Model file for the job. Use its own axes, mm. Face numbers are marked on the shaded views. A direction names the side the tool comes from. Round coordinates to 2 decimals unless told otherwise and drop trailing zeros. Loops run counter-clockwise (first coordinate to the right, second up) from the corner with the lowest first, then second, coordinate; pieces in that order, holes last. Notation, with made-up numbers: M -13.5,15.25 L 27.5,15.25 A24 cw 27.5,44.25 Z; hole C 4,50.25 d2. An arc over 180 degrees is marked long. Use a Markdown table: item, result. Add a question column.
Item 1: Saw through at D-D on z = 3.25. Write the cut outline in (x, y).
Item 2: Tool access for the marked faces 1, 2, 3, 4 and 5: list every direction of +Z, -Z, +X, -X, +Y, -Y with a clear straight run to the whole face (end or side of a thin tool).
Item 3: Wall check: L1, parallel to Y at x = -1.25, z = 0; L2, parallel to Y at x = 3, z = 0; L3, parallel to Z at x = 5, y = -4.25. Give the ranges that are in metal, low to high. Write a range as from..to.
Item 4: Saw through at A-A on z = 0. Write the cut outline in (x, y).
Item 5: Two-plate mould, pull along Y, no slides. Class the marked faces 6, 7 and 8: +Y half, -Y half, draft (parallel to the pull), parting line (faces both ways), or undercut.
Item 6: Saw through at B-B on y = 0. Write the cut outline in (x, z).
Item 7: Pin check, flat tips, straight feed: P1, Ø3, axis at y = -2, z = 7, coming from the -X side; P2, Ø6, axis at x = -1.5, z = 4, coming from the -Y side; P3, Ø6, axis at x = -4.5, y = -0.5, coming from the -Z side. Stop position of each tip, or through.
Item 8: Saw through at C-C on x = 9.25. Write the cut outline in (y, z).
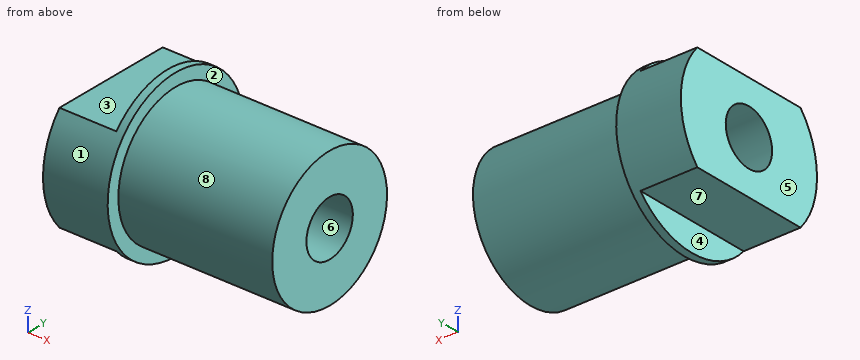
```python
from build123d import *

# Parameters (mm, degrees)
SKETCH2_R               = 7.9375
BOSS_EXTRUDE1_DEPTH     = 6.35
SKETCH3_R               = 6.6929
BOSS_EXTRUDE2_DEPTH     = 15.113
SKETCH4_W               = 5.588
SKETCH4_H               = 2.76225
CUT_EXTRUDE1_DEPTH      = 6.35
F_1_4_28_TAPPED_HOLE1_D = 5.4102


with BuildPart() as part:
    # Sketch2 → Boss-Extrude1 (new body)
    with BuildSketch(Plane(origin=(0, 0, 0), x_dir=(0, 0, -1), z_dir=(1, 0, 0))):
        Circle(SKETCH2_R)
    extrude(amount=-BOSS_EXTRUDE1_DEPTH)

    # Sketch3 → Boss-Extrude2 (add)
    with BuildSketch(Plane(origin=(0, 0, 0), x_dir=(0, 0, -1), z_dir=(1, 0, 0))):
        Circle(SKETCH3_R)
    extrude(amount=BOSS_EXTRUDE2_DEPTH)

    # Sketch4 → Cut-Extrude1 (cut, symmetric)
    with BuildSketch(Plane(origin=(0, 0, 0), x_dir=(1, 0, 0), z_dir=(0, 1, 0))):
        with Locations((-3.556, 6.556375)):
            Rectangle(SKETCH4_W, SKETCH4_H)
        with Locations((-3.556, -6.556375)):
            Rectangle(SKETCH4_W, SKETCH4_H)
    extrude(amount=CUT_EXTRUDE1_DEPTH, both=True, mode=Mode.SUBTRACT)

    # 1/4-28 Tapped Hole1 (through all)
    with Locations(Plane(origin=(-6.35, 0, 0), x_dir=(0, 0, -1), z_dir=(-1, 0, 0))):
        with Locations((0, 0)):
            Hole(F_1_4_28_TAPPED_HOLE1_D / 2)


solid = part.part
```
Entries:
| question | item | result |
|---|---|---|
| 1 | outline | M -6.35,-7.24 L 0,-7.24 L 0,-5.85 L 15.11,-5.85 L 15.11,5.85 L 0,5.85 L 0,7.24 L -6.35,7.24 Z |
| 2 | face 1 | +X, -X |
| 2 | face 2 | +X |
| 2 | face 3 | +Z, -X, +Y, -Y |
| 2 | face 4 | -Z, -X, +Y, -Y |
| 2 | face 5 | +Z, -Z, -X, +Y, -Y |
| 3 | L1 | -7.94..-2.71, 2.71..7.94 |
| 3 | L2 | -6.69..-2.71, 2.71..6.69 |
| 3 | L3 | -5.17..5.17 |
| 4 | outline | M -6.35,-7.94 L 0,-7.94 L 0,-6.69 L 15.11,-6.69 L 15.11,-2.71 L -6.35,-2.71 Z; M -6.35,2.71 L 15.11,2.71 L 15.11,6.69 L 0,6.69 L 0,7.94 L -6.35,7.94 Z |
| 5 | face 6 | undercut |
| 5 | face 7 | draft |
| 5 | face 8 | parting line |
| 6 | outline | M -6.35,-5.18 L -0.76,-5.18 L -0.76,-7.94 L 0,-7.94 L 0,-6.69 L 15.11,-6.69 L 15.11,-2.71 L -6.35,-2.71 Z; M -6.35,2.71 L 15.11,2.71 L 15.11,6.69 L 0,6.69 L 0,7.94 L -0.76,7.94 L -0.76,5.18 L -6.35,5.18 Z |
| 7 | P1 | x = -0.76 |
| 7 | P2 | y = -7.87 |
| 7 | P3 | z = -5.18 |
| 8 | outline | C 0,0 d13.39; hole C 0,0 d5.41 |
